Can you work these out from the model? Positions are in its coordinate system, mm. Face numbers are marked on the shaded views. A direction names the side the tool comes from. Round coordinates to 2 decimals unless told otherwise and drop trailing zeros. Write each loop counter-clockwise with the first axis right and the second up, starting at its lowest first coordinate (ties: lowest second). Pieces come first, ordered by that corner, then holes. Notation, with made-up numbers: (57, 4) - (98, 4) arc R22 ccw to (98, 38) - close; hole circle Ø9 at (-39.5, -17.75). An arc over 180 degrees is marked (long way). One line per item, written item: value. Start each with the question number.
(1) I want a section at A-A on y = -13.5. List the corners of the cut face in (x, z) for me (3 decimals).
(2) On a 3-axis mill with a long thin cutter (end or side, diameter ignored), from which of +Z, -Z, +X, -X, +Y, -Y can I reach the whole of each face in a straight line? I mean the marked faces 1 and 2. Say none if no direction works.
(3) I want a section at B-B on x = -36.5. List the corners of the cut face in (y, z) for me (3 decimals), plus the area to 3 significant figures.
(4) I'm going to push flat-ended pins straight in: pin 1 Ø3 at (y, z) = (-14, -0.5) entering from -X; pin 2 Ø2 at (x, z) = (-33.5, 4.5) entering from -Y. Where does each tip first touch, or does it pass through?
(5) I want a section at C-C on y = 3. List the corners of the cut face in (x, z) for me.
(6) If I drill on L1, parallel to Y at x = -37.5, z = 0 (3 decimals); L2, parallel to Y at x = -39.25, z = 0 (3 decimals); L3, parallel to X at y = -1, z = 4, over which ranges is the centre line in solid material (lowest first)? Write a range as from..to.
(7) Thinking about a two-plate mould opening in X: for the marked faces 3, 4, 5 and 6, which applies, +X half, -X half, draft (parallel to the pull), parting line (faces both ways), or undercut?
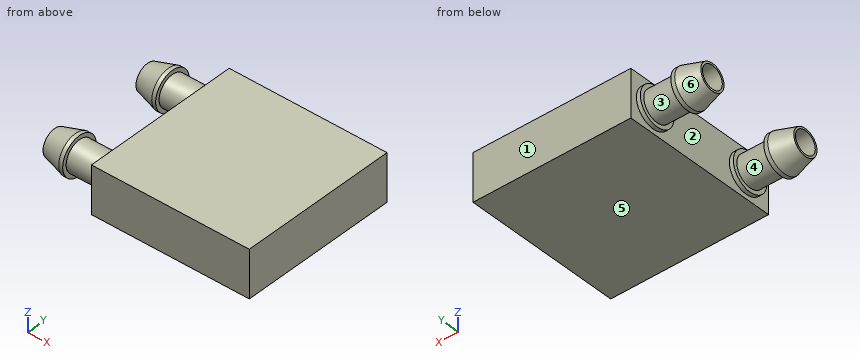
from build123d import *

# Parameters (mm, degrees)
BOSS_EXTRUDE_BASE_DEPTH      = 6
BOSS_EXTRUDE_BASE_DEPTH_BACK = 6
BASE_W                       = 40.00000001
BASE_H                       = 40


with BuildPart() as part:
    # Base → Boss-Extrude Base (new, two sides: drawn at the far end of the back side and taken through both)
    with BuildSketch(Plane.XY.offset(-BOSS_EXTRUDE_BASE_DEPTH_BACK)):
        with Locations((-10, 0)):
            Rectangle(BASE_W, BASE_H)
    extrude(amount=BOSS_EXTRUDE_BASE_DEPTH + BOSS_EXTRUDE_BASE_DEPTH_BACK)

    # Port Profile → Revolve Port (revolve)
    with BuildSketch(Plane.XY, mode=Mode.PRIVATE) as revolve_port_sk:
        Polygon((-30.000000005, 16.375000092), (-45.000000005, 16.375000092), (-45.000000005, 16.875000092), (-39.700000005, 18.375000092), (-38.700000005, 18.375000092), (-38.700000005, 17.375000092), (-31.000000037, 17.375000092), (-31.000000037, 18.375000092), (-30.000000005, 18.375000092), align=None)
    revolve_port = revolve(revolve_port_sk.sketch.rotate(Axis((-30, 13.5, 0), (-1, 0, 0)), 90), axis=Axis((-30, 13.5, 0), (-1, 0, 0)))

    # Mirror Port: Revolve Port across plane
    add(revolve_port.mirror(Plane.ZX))


solid = part.part
Established:
1. outline: (-45, -3.375) - (-39.7, -4.875) - (-38.7, -4.875) - (-38.7, -3.875) - (-31, -3.875) - (-31, -4.875) - (-30, -4.875) - (-30, -6) - (10, -6) - (10, 6) - (-30, 6) - (-30, 4.875) - (-31, 4.875) - (-31, 3.875) - (-38.7, 3.875) - (-38.7, 4.875) - (-39.7, 4.875) - (-45, 3.375) - (-45, 2.875) - (-30, 2.875) - (-30, -2.875) - (-45, -2.875) - close
2. face 1: +Z, -Z, +X, -X, +Y
2. face 2: -X
3. outline: circle Ø7.75 at (-13.5, 0); circle Ø7.75 at (13.5, 0); hole circle Ø5.75 at (-13.5, 0); hole circle Ø5.75 at (13.5, 0)
3. area: 42.4 mm2
4. pin 1: x = -30
4. pin 2: y = -15.16
5. outline: (-30, -6) - (10, -6) - (10, 6) - (-30, 6) - close
6. L1: -17.375..-16.375, -10.625..-9.625, 9.625..10.625, 16.375..17.375
6. L2: -18.375..-16.375, -10.625..-8.625, 8.625..10.625, 16.375..18.375
6. L3: -30..10
7. face 3: undercut
7. face 4: undercut
7. face 5: draft
7. face 6: -X half
